from build123d import *

# Parameters (mm, degrees)
ESQUISSE1_W             = 15
ESQUISSE1_H             = 15
EXTRUSION1_DEPTH        = 80
ESQUISSE2_W             = 12
ESQUISSE2_H             = 12
EXTRUSION2_DEPTH        = 81.700061958
ESQUISSE3_R             = 1.5
ENL_V_MAT_EXTRU_1_DEPTH = 82.738913621


with BuildPart() as part:
    # Esquisse1 → Extrusion1 (new body)
    with BuildSketch(Plane.XY):
        Rectangle(ESQUISSE1_W, ESQUISSE1_H)
    extrude(amount=EXTRUSION1_DEPTH)

    # Esquisse2 → Extrusion2 (cut, through all)
    with BuildSketch(Plane.XY.offset(80)):
        Rectangle(ESQUISSE2_W, ESQUISSE2_H)
    extrude(amount=-EXTRUSION2_DEPTH, mode=Mode.SUBTRACT)

    # Esquisse3 → Enlèv. mat.-Extru.1 (cut, through all)
    with BuildSketch(Plane(origin=(7.5, 0, 0), x_dir=(0, 0, -1), z_dir=(1, 0, 0))):
        with Locations((-5, 0)):
            Circle(ESQUISSE3_R)
        with Locations((-15, 0)):
            Circle(ESQUISSE3_R)
    extrude(amount=-ENL_V_MAT_EXTRU_1_DEPTH, mode=Mode.SUBTRACT)


solid = part.part
Part model, mm, in its own coordinate system. A direction names the side the tool comes from. Round coordinates to 2 decimals unless told otherwise and drop trailing zeros. Loops run counter-clockwise (first coordinate to the right, second up) from the corner with the lowest first, then second, coordinate; pieces in that order, holes last. Notation, with made-up numbers: (-13, 36) - (8, 36) arc R23 cw to (8, 61) - close; hole circle Ø8 at (58.5, 13). An arc over 180 degrees is marked (long way). Answer as a JSON object with one key per item and string values.
Item 1: Pull direction X, two halves, no side cores. Call faces 1 (the face through (0, -6, 41)), 2 (the face through (-7.5, 0, 39)), 3 (the face through (-6.74, 0.07, 16.5)): pulls with the +X half, pulls with the -X half, needs draft (parallel to the pull), parting line crosses it, or undercut.
Output:
{"face 1": "undercut", "face 2": "pulls with the -X half", "face 3": "needs draft"}
Item 2: Tool access for faces 4 (the face through (6.8, -0.9, 6.2)), 5 (the face through (0, 6, 41)): list every direction of +Z, -Z, +X, -X, +Y, -Y with a clear straight run to the whole face (end or side of a thin tool).
Output:
{"face 4": "+X, -X", "face 5": "+Z, -Z"}
Item 3: Pin check, flat tip, straight feed: pin 1 (6 mm diameter, centred on x = -4.5, y = -0.5, fed in from -Z). Stop position of the tip, or through.
Output:
{"pin 1": "z = 0"}
Item 4: Band-saw the part on D-D on z = 5. List the corners of the cut face in (x, y), plus the area to 3 significant figures.
Output:
{"outline": "(-7.5, -7.5) - (7.5, -7.5) - (7.5, -1.5) - (6, -1.5) - (6, -6) - (-6, -6) - (-6, -1.5) - (-7.5, -1.5) - close; (-7.5, 1.5) - (-6, 1.5) - (-6, 6) - (6, 6) - (6, 1.5) - (7.5, 1.5) - (7.5, 7.5) - (-7.5, 7.5) - close", "area": "72.0 mm2"}
Item 5: Band-saw the part on B-B on z = 52. List the corners of the cut face in (x, y), plus the area to 3 significant figures.
Output:
{"outline": "(-7.5, -7.5) - (7.5, -7.5) - (7.5, 7.5) - (-7.5, 7.5) - close; hole (-6, -6) - (6, -6) - (6, 6) - (-6, 6) - close", "area": "81.0 mm2"}
Item 6: Wall check: L1, parallel to Y at x = -6.6, z = 5; L2, parallel to X at y = -1, z = 27. Give the ranges that are in metal, low to high.
Output:
{"L1": "-7.5 to -1.5, 1.5 to 7.5", "L2": "-7.5 to -6, 6 to 7.5"}
Item 7: Band-saw the part on C-C on y = 0. List the corners of the cut face in (x, z).
Output:
{"outline": "(-7.5, 0) - (-6, 0) - (-6, 3.5) - (-7.5, 3.5) - close; (-7.5, 6.5) - (-6, 6.5) - (-6, 13.5) - (-7.5, 13.5) - close; (-7.5, 16.5) - (-6, 16.5) - (-6, 80) - (-7.5, 80) - close; (6, 0) - (7.5, 0) - (7.5, 3.5) - (6, 3.5) - close; (6, 6.5) - (7.5, 6.5) - (7.5, 13.5) - (6, 13.5) - close; (6, 16.5) - (7.5, 16.5) - (7.5, 80) - (6, 80) - close"}
Item 8: Band-saw the part on A-A on x = -3.75. List the corners of the cut face in (y, z), plus the area to 3 significant figures.
Output:
{"outline": "(-7.5, 0) - (-6, 0) - (-6, 80) - (-7.5, 80) - close; (6, 0) - (7.5, 0) - (7.5, 80) - (6, 80) - close", "area": "240 mm2"}
